```python
from build123d import *

# Parameters (mm, degrees)
SKETCH1_W           = 120
SKETCH1_H           = 55
SKETCH1_R           = 2
BOSS_EXTRUDE1_DEPTH = 1.5


with BuildPart() as part:
    # Sketch1 → Boss-Extrude1 (new body, symmetric)
    with BuildSketch(Plane.XY):
        Rectangle(SKETCH1_W, SKETCH1_H)
        with Locations((-15, 0)):
            Circle(SKETCH1_R, mode=Mode.SUBTRACT)
        with Locations((15, 0)):
            Circle(SKETCH1_R, mode=Mode.SUBTRACT)
        with Locations((15, -15)):
            Circle(SKETCH1_R, mode=Mode.SUBTRACT)
        with Locations((-15, -15)):
            Circle(SKETCH1_R, mode=Mode.SUBTRACT)
        with BuildLine():
            Line((-50, 22.5), (50, 22.5))
            ThreePointArc((50, 22.5), (52.5, 20), (50, 17.5))
            Line((50, 17.5), (-50, 17.5))
            ThreePointArc((-50, 17.5), (-52.5, 20), (-50, 22.5))
        make_face(mode=Mode.SUBTRACT)
    extrude(amount=BOSS_EXTRUDE1_DEPTH, both=True)


solid = part.part
```
Input: part model. Units: mm. Frame: model coordinates. A direction names the side the tool comes from. Give positions to 0.01 mm unless a question says otherwise; leave off trailing zeros. Order: outer loops, then holes, each group sorted by start corner. A loop starts at its lowest first (then second) coordinate and runs counter-clockwise, first axis right, second up. Notation, with made-up numbers: M -32.5,-31 L -9.5,-31 A27 ccw -9.5,-8 Z; hole C 17.5,66.25 d2. An arc over 180 degrees is marked long. Return JSON: item names as keys, results as strings.
Item 1: Cut plane D-D (x = -15). Return loops of the section in (y, z).
Solutions:
{"outline": "M -27.5,-1.5 L -17,-1.5 L -17,1.5 L -27.5,1.5 Z; M -13,-1.5 L -2,-1.5 L -2,1.5 L -13,1.5 Z; M 2,-1.5 L 17.5,-1.5 L 17.5,1.5 L 2,1.5 Z; M 22.5,-1.5 L 27.5,-1.5 L 27.5,1.5 L 22.5,1.5 Z"}
Item 2: Pull-direction query (X, two-part tool) for faces 1 (the flat face through (-60, 0, 0)), 2 (the flat face through (1, 17.5, 0)), 3 (the flat face through (-1, 27.5, 0)), 4 (the flat face through (60, 0, 0)); classes: +X half, -X half, draft (parallel to the pull), parting line (faces both ways), or undercut.
Solutions:
{"face 1": "-X half", "face 2": "undercut", "face 3": "draft", "face 4": "+X half"}
Item 3: Cut plane C-C (x = -27). Return loops of the section in (y, z).
Solutions:
{"outline": "M -27.5,-1.5 L 17.5,-1.5 L 17.5,1.5 L -27.5,1.5 Z; M 22.5,-1.5 L 27.5,-1.5 L 27.5,1.5 L 22.5,1.5 Z"}
Item 4: Cut plane B-B (z = 0). Return loops of the section in (x, y), then the cut area to 3 significant figures.
Solutions:
{"outline": "M -60,-27.5 L 60,-27.5 L 60,27.5 L -60,27.5 Z; hole M -50,17.5 L 50,17.5 A2.5 ccw 50,22.5 L -50,22.5 A2.5 ccw Z; hole C -15,-15 d4; hole C -15,0 d4; hole C 15,-15 d4; hole C 15,0 d4", "area": "6,030 mm^2"}
Item 5: Access query for faces 5 (the cylindrical face through (-52.5, 19.9, 0)), 6 (the flat face through (-1, 0, 1.5)). Directions: +Z, -Z, +X, -X, +Y, -Y. A direction counts if a zero-diameter tool reaches every point of the face in a straight line with its end or side. Return the directions, or none.
Solutions:
{"face 5": "+Z, -Z", "face 6": "+Z, +X, -X, +Y, -Y"}
Item 6: Cut plane A-A (y = 0). Return loops of the section in (x, z).
Solutions:
{"outline": "M -60,-1.5 L -17,-1.5 L -17,1.5 L -60,1.5 Z; M -13,-1.5 L 13,-1.5 L 13,1.5 L -13,1.5 Z; M 17,-1.5 L 60,-1.5 L 60,1.5 L 17,1.5 Z"}
Item 7: Ray query, probe 1 along Y at (x, z) = (-15, -0.65); probe 2 along Y at (x, z) = (-36, -0.8); probe 3 along X at (y, z) = (-13.5, -0.7). Return the intervals inside material, ascending.
Solutions:
{"probe 1": "-27.5 to -17, -13 to -2, 2 to 17.5, 22.5 to 27.5", "probe 2": "-27.5 to 17.5, 22.5 to 27.5", "probe 3": "-60 to -16.32, -13.68 to 13.68, 16.32 to 60"}
